Part model, mm, in its own coordinate system. A direction names the side the tool comes from. Round coordinates to 2 decimals unless told otherwise and drop trailing zeros. Loops run counter-clockwise (first coordinate to the right, second up) from the corner with the lowest first, then second, coordinate; pieces in that order, holes last.
(1) Cut at D-D on x = -16.5. List the corners of the cut face in (y, z).
(2) Cut at B-B on z = 20.5. List the corners of the cut face in (x, y), then the cut area to 3 significant figures.
(3) Probe probe 1 along Y at (x, z) = (-13, 23); probe 2 along Y at (x, z) = (16.5, 23.5); probe 3 along Z at (x, y) = (14, -40) (3 decimals). List the from-to ranges inside material, lowest first.
(4) Flat gauge pins, fed straight in: pin 1 (10 mm diameter, centred on x = -5.5, z = 37, fed in from +Y); pin 2 (5 mm diameter, centred on x = 4.5, y = -15, fed in from +Z); pin 3 (10 mm diameter, centred on x = 0, y = -17.5, fed in from -Z); pin 4 (2.5 mm diameter, centred on x = 14.5, y = -41, fed in from -Z). Where does each tip first touch, or does it go through?
(5) Tool access for faces 1 (the face through (1, -45, 31)), 2 (the face through (7, -15, 16)), 3 (the face through (-25, -30, 25)), 4 (the face through (1, -41, 18)): list every direction of +Z, -Z, +X, -X, +Y, -Y with a clear straight run to the whole face (end or side of a thin tool).
(6) Cut at C-C on y = -9. List the corners of the cut face in (x, z).
(7) Cut at A-A on x = -1. List the corners of the cut face in (y, z).
from build123d import *

# Parameters (mm, degrees)
BOSS_EXTRUDE3_DEPTH = 40
CUT_EXTRUDE1_DEPTH  = 51
CUT_EXTRUDE3_DEPTH  = 51


with BuildPart() as part:
    # Sketch8 → Boss-Extrude3 (new body, symmetric)
    with BuildSketch(Plane(origin=(0, 0, 0), x_dir=(0, 0, -1), z_dir=(1, 0, 0))):
        Polygon((-50, -30), (-50, -37), (-43, -45), (-18, -45), (-18, -37), (0, -37), (0, 0), (-8.660254038, -15), (-24.019237886, -15), align=None)
    extrude(amount=BOSS_EXTRUDE3_DEPTH, both=True)

    # Sketch10 → Cut-Extrude1 (cut, through all)
    with BuildSketch(Plane.XY.offset(50)):
        Polygon((-10, 0), (-40, 0), (-40, -15), (-40, -30), (-10, -30), align=None)
    extrude(amount=-CUT_EXTRUDE1_DEPTH, mode=Mode.SUBTRACT)

    # Sketch11 → Cut-Extrude3 (cut, through all)
    with BuildSketch(Plane.XY.offset(50)):
        Polygon((40, 0), (15, 0), (23.333333333, -15), (40, -15), align=None)
        Polygon((40, -15), (23.333333333, -15), (40, -45), (40, -37), (40, -30), align=None)
    extrude(amount=-CUT_EXTRUDE3_DEPTH, mode=Mode.SUBTRACT)


solid = part.part
Final values:
1. outline: (-45, 18) - (-37, 18) - (-37, 0) - (-30, 0) - (-30, 50) - (-37, 50) - (-45, 43) - close
2. outline: (-40, -45) - (40, -45) - (23.33, -15) - (-10, -15) - (-10, -30) - (-40, -30) - close
2. area: 1,700 mm2
3. probe 1: y = -45 to -30
3. probe 2: y = -45 to -15
3. probe 3: z = 18 to 47.375
4. pin 1: stops at y = -19.61
4. pin 2: stops at z = 28.35
4. pin 3: stops at z = 0
4. pin 4: stops at z = 18
5. face 1: +Z, -Z, +X, -X, -Y
5. face 2: +Z, +X, -X, +Y
5. face 3: +Z, -Z, -X, +Y
5. face 4: -Z, +X, -X, -Y
6. outline: (-10, 0) - (20, 0) - (20, 5.2) - (-10, 5.2) - close
7. outline: (-45, 18) - (-37, 18) - (-37, 0) - (0, 0) - (-15, 8.66) - (-15, 24.02) - (-30, 50) - (-37, 50) - (-45, 43) - close
